The model under review builds one solid part; all positions refer to its coordinate system, in mm. A direction names the side the tool comes from. Round coordinates to 2 decimals unless told otherwise and drop trailing zeros. Order: outer loops, then holes, each group sorted by start corner. A loop starts at its lowest first (then second) coordinate and runs counter-clockwise, first axis right, second up. Notation, with made-up numbers: M -23,-22.5 L 9,-22.5 A29 ccw 9,14.5 Z; hole C 39.5,-31 d2. An arc over 180 degrees is marked long. Answer as a JSON object with one key per item and string values. Group by question number.
1. Add section A-A on z = -8. State the section outline as (x, y) points, and give its area (3 significant figures).
2. To check wall thickness, follow probe 1 along Z at (x, y) = (4.55, 2.9); probe 2 along X at (y, z) = (2.05, -8); probe 3 along Y at (x, z) = (14.25, -3.75). State the ranges of each line that lie inside material, in increasing order. Write a range as [from, to].
3. Add section C-C on y = 1.35. State the section outline as (x, z) points, and give its area (3 significant figures).
4. Add section B-B on x = 4.55. State the section outline as (y, z) points, and give its area (3 significant figures).
5. Clearance check with a flat-ended pin moving along its axis: P1, Ø3, axis at x = 15.5, z = -8, coming from the +Y side. State where the tip first meets the part, or that it passes through.
6. Add section D-D on z = -12.25. State the section outline as (x, y) points.
7. Machinability: for faces 1 (the face through (-2.5, 1.8, -8.1)), 2 (the face through (3.54, 4.67, -3.46)), which of the approach directions +Z, -Z, +X, -X, +Y, -Y give a long, thin tool a straight path to every point of the face, cutting with its end or side? Answer none if there is none.
```python
from build123d import *

# Parameters (mm, degrees)
SKETCH2_R           = 3.96875
BOSS_EXTRUDE1_DEPTH = 3.68
SKETCH3_R           = 4.65
SKETCH3_R_2         = 3.96875
BOSS_EXTRUDE2_DEPTH = 2


with BuildPart() as part:
    # Sketch2 → Boss-Extrude1 (new body)
    with BuildSketch(Plane(origin=(0, 0, 0), x_dir=(1, 0, 0), z_dir=(0, 1, 0))):
        with BuildLine():
            Line((0, 0), (20, 0))
            ThreePointArc((20, 0), (22.5, 8), (20, 16))
            Line((20, 16), (0, 16))
            ThreePointArc((0, 16), (-2.5, 8), (0, 0))
        make_face()
        with Locations((4.55, 8)):
            Circle(SKETCH2_R, mode=Mode.SUBTRACT)
    extrude(amount=BOSS_EXTRUDE1_DEPTH)

    # Sketch3 → Boss-Extrude2 (add)
    with BuildSketch(Plane(origin=(0, 3.68, 0), x_dir=(1, 0, 0), z_dir=(0, 1, 0))):
        with Locations((4.55, 8)):
            Circle(SKETCH3_R)
        with Locations((4.55, 8)):
            Circle(SKETCH3_R_2, mode=Mode.SUBTRACT)
    extrude(amount=BOSS_EXTRUDE2_DEPTH)


solid = part.part
```
Recorded:
{
 "1": {"outline": "M -2.5,0 L 0.58,0 L 0.58,5.68 L -0.1,5.68 L -0.1,3.68 L -2.5,3.68 Z; M 8.52,0 L 22.5,0 L 22.5,3.68 L 9.2,3.68 L 9.2,5.68 L 8.52,5.68 Z", "area": "65.5 mm²"},
 "2": {"probe 1": "z = [-16, -11.97], [-4.03, 0]", "probe 2": "x = [-2.5, 0.58], [8.52, 22.5]", "probe 3": "y = [0, 3.68]"},
 "3": {"outline": "M 0,-16 L 20,-16 A14.05 ccw 20,0 L 0,0 A14.05 ccw Z; hole C 4.55,-8 d7.94", "area": "325 mm²"},
 "4": {"outline": "M 0,-16 L 3.68,-16 L 3.68,-12.65 L 5.68,-12.65 L 5.68,-11.97 L 0,-11.97 Z; M 0,-4.03 L 5.68,-4.03 L 5.68,-3.35 L 3.68,-3.35 L 3.68,0 L 0,0 Z", "area": "32.4 mm²"},
 "5": {"P1": "stops at y = 3.68"},
 "6": {"outline": "M -1.84,0 L 21.84,0 L 21.84,3.68 L 6.44,3.68 L 6.44,5.68 L 2.66,5.68 L 2.66,3.68 L -1.84,3.68 Z"},
 "7": {"face 1": "-X, +Y, -Y", "face 2": "+Y"}
}
